```python
from build123d import *

# Parameters (mm, degrees)
SKETCH1_R           = 15
SKETCH1_R_2         = 7.5
BOSS_EXTRUDE1_DEPTH = 1


with BuildPart() as part:
    # Sketch1 → Boss-Extrude1 (new body)
    with BuildSketch(Plane.XY):
        with BuildLine():
            Line((-15.701917229, 8.165829146), (-15.701917229, 33.165829146))
            Line((-15.701917229, 33.165829146), (14.298082771, 33.165829146))
            Line((14.298082771, 33.165829146), (14.298082771, 8.165829146))
            Line((14.298082771, 8.165829146), (39.298082771, 8.165829146))
            ThreePointArc((39.298082771, 8.165829146), (46.369150582, 5.236896958), (49.298082771, -1.834170854))
            Line((49.298082771, -1.834170854), (49.298082771, -26.834170854))
            ThreePointArc((49.298082771, -26.834170854), (46.369150582, -33.905238666), (39.298082771, -36.834170854))
            Line((39.298082771, -36.834170854), (-40.701917229, -36.834170854))
            ThreePointArc((-40.701917229, -36.834170854), (-47.772985041, -33.905238666), (-50.701917229, -26.834170854))
            Line((-50.701917229, -26.834170854), (-50.701917229, -1.834170854))
            ThreePointArc((-50.701917229, -1.834170854), (-47.772985041, 5.236896958), (-40.701917229, 8.165829146))
            Line((-40.701917229, 8.165829146), (-15.701917229, 8.165829146))
        make_face()
        with Locations((-10.701917229, -16.834170854)):
            Circle(SKETCH1_R, mode=Mode.SUBTRACT)
        with Locations((24.298082771, -6.834170854)):
            Circle(SKETCH1_R_2, mode=Mode.SUBTRACT)
    extrude(amount=BOSS_EXTRUDE1_DEPTH)


solid = part.part
```
Can you work these out from the model? Positions are in its coordinate system, mm. Coordinates: 2 decimals unless noted, no trailing zeros. Loops run counter-clockwise (first coordinate to the right, second up) from the corner with the lowest first, then second, coordinate; pieces in that order, holes last. Notation, with made-up numbers: M -29.5,32 L 20.5,32 A26 cw 20.5,54 Z; hole C 30.25,-8 d7. An arc over 180 degrees is marked long. Put each result on its own line as item: value. Start each with the question number.
(1) We'd pull the mould along Y, two halves only. Please class faces 1 (the face through (46.446, -33.827, 0.493)), 2 (the face through (-2.638, -4.186, 0.493)), 3 (the face through (0, -1, 0)): +Y half, -Y half, draft (parallel to the pull), parting line (faces both ways), or undercut.
(2) Imagine slicing it at B-B on y = -0.5. List the corners of the cut face in (x, z) for me.
(3) Imagine slicing it at A-A on x = 1.5. List the corners of the cut face in (y, z) for me, and give its area (3 significant figures).
(4) I need wall thicknesses on probe 1 along X at (y, z) = (24, 0.8); probe 2 along X at (y, z) = (-14.5, 0.75); probe 3 along X at (y, z) = (-27.5, 0.2). Which ranges of each line are inside material? Lowest first, please.
(5) Imagine slicing it at D-D on y = -10. List the corners of the cut face in (x, z) for me, and give its area (3 significant figures).
(6) Imagine slicing it at C-C on z = 0.4. List the corners of the cut face in (x, y) for me.
Worked answers:
1. face 1: -Y half
1. face 2: undercut
1. face 3: draft
2. outline: M -50.61,0 L 20.28,0 L 20.28,1 L -50.61,1 Z; M 28.31,0 L 49.21,0 L 49.21,1 L 28.31,1 Z
3. outline: M -36.83,0 L -25.56,0 L -25.56,1 L -36.83,1 Z; M -8.11,0 L 33.17,0 L 33.17,1 L -8.11,1 Z
3. area: 52.6 mm2
4. probe 1: x = -15.7 to 14.3
4. probe 2: x = -50.7 to -25.52, 4.12 to 49.3
4. probe 3: x = -50.68 to -21.25, -0.15 to 49.28
5. outline: M -50.7,0 L -24.05,0 L -24.05,1 L -50.7,1 Z; M 2.65,0 L 17.5,0 L 17.5,1 L 2.65,1 Z; M 31.1,0 L 49.3,0 L 49.3,1 L 31.1,1 Z
5. area: 59.7 mm2
6. outline: M -50.7,-26.83 A10 ccw -40.7,-36.83 L 39.3,-36.83 A10 ccw 49.3,-26.83 L 49.3,-1.83 A10 ccw 39.3,8.17 L 14.3,8.17 L 14.3,33.17 L -15.7,33.17 L -15.7,8.17 L -40.7,8.17 A10 ccw -50.7,-1.83 Z; hole C -10.7,-16.83 d30; hole C 24.3,-6.83 d15
